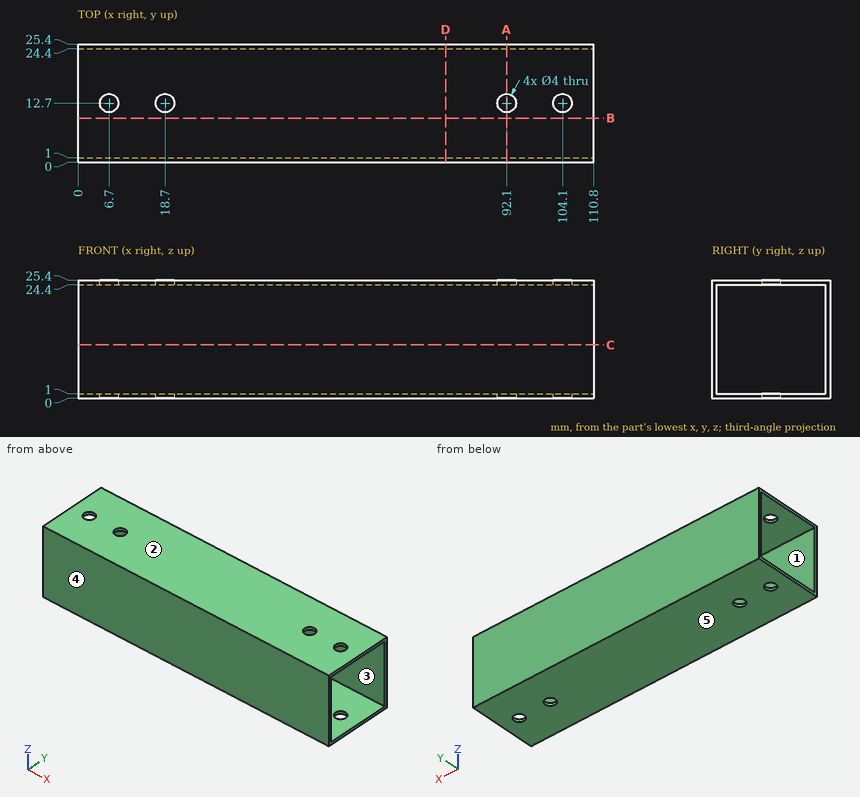
Answer from the drawing. Dimensions are ordinates in mm from the lowest x, y and z of the part. A direction names the side the tool comes from. Round coordinates to 2 decimals unless told otherwise and drop trailing zeros. Write each loop counter-clockwise with the first axis right and the second up, starting at its lowest first coordinate (ties: lowest second). Pieces come first, ordered by that corner, then holes.
1. The part is cut by section B-B, the plane y = 9.5. Determine the outline of the cut face in (x, z), then the cut area to 3 significant figures.
2. The part is cut by section D-D, the plane x = 79. Determine the outline of the cut face in (y, z).
3. Straight lines are drawn through the part: L1, parallel to Y at x = 34.5, z = 5.5; L2, parallel to Y at x = 104.1, z = 0.55. For each, find the intervals that lie inside material, in ascending order.
4. Determine the mould class of the marked faces 3, 4 and 5 for opening direction Y: pulls with the +Y half, pulls with the -Y half, needs draft (parallel to the pull), parting line crosses it, or undercut.
5. Which of the six approach directions +Z, -Z, +X, -X, +Y, -Y give full straight-line access (tool end or side, diameter ignored) to the marked faces 1 and 2?
6. The part is cut by section A-A, the plane x = 92.1. Determine the outline of the cut face in (y, z).
7. Given pin 1 Ø2.5 at (x, y) = (92.1, 12.7) entering from +Z, flat-ended and moving along its own axis, determine where the tip first touches the part or whether it passes through.
Values:
1. outline: (0, 0) - (110.8, 0) - (110.8, 1) - (0, 1) - close; (0, 24.4) - (110.8, 24.4) - (110.8, 25.4) - (0, 25.4) - close
1. area: 222 mm2
2. outline: (0, 0) - (25.4, 0) - (25.4, 25.4) - (0, 25.4) - close; hole (1, 1) - (24.4, 1) - (24.4, 24.4) - (1, 24.4) - close
3. L1: y = 0 to 1, 24.4 to 25.4
3. L2: y = 0 to 10.7, 14.7 to 25.4
4. face 3: undercut
4. face 4: pulls with the -Y half
4. face 5: needs draft
5. face 1: +X, -X
5. face 2: +Z, +X, -X, +Y, -Y
6. outline: (0, 0) - (10.7, 0) - (10.7, 1) - (1, 1) - (1, 24.4) - (10.7, 24.4) - (10.7, 25.4) - (0, 25.4) - close; (14.7, 0) - (25.4, 0) - (25.4, 25.4) - (14.7, 25.4) - (14.7, 24.4) - (24.4, 24.4) - (24.4, 1) - (14.7, 1) - close
7. pin 1: passes through
